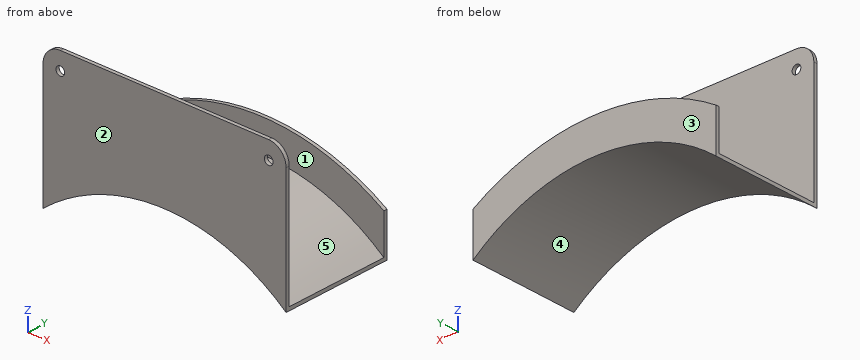
```python
from build123d import *

# Parameters (mm, degrees)
F1_DEPTH = 1.27
F3_DEPTH = 38.1
F5_DEPTH = 1.27
F6_R     = 1.5875
F7_DEPTH = 25.4


with BuildPart() as f1:
    # F0 (on Front) → F1 (new body)
    with BuildSketch(Plane.XZ):
        with BuildLine():
            Line((-44.45, 15.644758), (-44.45, 0))
            ThreePointArc((-44.45, 0), (0, 15.875), (44.45, 0))
            Line((44.45, 0), (44.45, 15.644758))
            ThreePointArc((44.45, 15.644758), (0, 28.575), (-44.45, 15.644758))
        make_face()
    extrude(amount=F1_DEPTH)

    # F2 (on face) → F3 (join)
    with BuildSketch(Plane.XZ.offset(1.27)):
        with BuildLine():
            ThreePointArc((-44.45, 0), (0, 15.875), (44.45, 0))
            Line((44.45, 0), (44.45, 1.27))
            ThreePointArc((44.45, 1.27), (0, 16.862218), (-44.45, 1.27))
            Line((-44.45, 1.27), (-44.45, 0))
        make_face()
    extrude(amount=F3_DEPTH)

    # F4 (on face) → F5 (join)
    with BuildSketch(Plane.XZ.offset(39.37)):
        with BuildLine():
            Line((-44.45, 44.45), (-44.45, 0))
            ThreePointArc((-44.45, 0), (0, 15.875), (44.45, 0))
            Line((44.45, 0), (44.45, 44.45))
            ThreePointArc((44.45, 44.45), (42.590128, 48.940128), (38.1, 50.8))
            Line((38.1, 50.8), (-38.1, 50.8))
            ThreePointArc((-38.1, 50.8), (-42.590128, 48.940128), (-44.45, 44.45))
        make_face()
    extrude(amount=F5_DEPTH)

    # F6 (on face) → F7 (cut)
    with BuildSketch(Plane(origin=(0, -39.37, 0), x_dir=(-1, 0, 0), z_dir=(0, 1, 0))):
        with Locations((-38.1, 44.45)):
            Circle(F6_R)
        with Locations((38.1, 44.45)):
            Circle(F6_R)
    extrude(amount=-F7_DEPTH, mode=Mode.SUBTRACT)


solid = f1.part
```
The model under review builds one solid part; all positions refer to its coordinate system, in mm. Face numbers are marked on the shaded views. A direction names the side the tool comes from. Round coordinates to 2 decimals unless told otherwise and drop trailing zeros. Write each loop counter-clockwise with the first axis right and the second up, starting at its lowest first coordinate (ties: lowest second). Pieces come first, ordered by that corner, then holes.
(1) We need section D-D on z = 18. Give the boundary of the cut face in (x, y).
(2) Machinability: for the marked faces 1 and 2, which of the approach directions +Z, -Z, +X, -X, +Y, -Y give a long, thin tool a straight path to every point of the face, cutting with its end or side? Answer none if there is none.
(3) We need section C-C on x = -30.5. Give the boundary of the cut face in (y, z).
(4) We need section A-A on z = 8. Give the boundary of the cut face in (x, y), and give its area (3 significant figures).
(5) Mouldability with a two-part tool opening along X and no side actions: class the marked faces 3, 4 and 5 as +X half, -X half, draft (parallel to the pull), parting line (faces both ways), or undercut.
(6) Wall thickness on L1, parallel to Y at x = 3.5, z = 22.5; L2, parallel to X at y = -40, z = 44; L3, parallel to Y at x = -22, z = 41: over which ranges is each line inside the solid? List them lowest first.
(7) Insertion check: pin 1 (5 mm diameter, centred on x = -38.1, z = 44.45, fed in from +Y); pin 2 (4 mm diameter, centred on x = -34.5, y = -25.5, fed in from -Z); pin 3 (5 mm diameter, centred on x = 21.5, y = -28.5, fed in from -Z). Each pin has a flat end and moves straight along its axis. Give the tip position at first contact, or say it passes through.
Findings below:
1. outline: (-44.45, -40.64) - (44.45, -40.64) - (44.45, -39.37) - (-44.45, -39.37) - close; (-40.51, -1.27) - (40.51, -1.27) - (40.51, 0) - (-40.51, 0) - close
2. face 1: +Z
2. face 2: +Z, -Z, +X, -X, -Y
3. outline: (-40.64, 8.9) - (0, 8.9) - (0, 22.76) - (-1.27, 22.76) - (-1.27, 9.99) - (-39.37, 9.99) - (-39.37, 50.8) - (-40.64, 50.8) - close
4. outline: (-44.45, -40.64) - (-32.3, -40.64) - (-32.3, 0) - (-44.45, 0) - (-44.45, -1.27) - (-34.39, -1.27) - (-34.39, -39.37) - (-44.45, -39.37) - close; (32.3, -40.64) - (44.45, -40.64) - (44.45, -39.37) - (34.39, -39.37) - (34.39, -1.27) - (44.45, -1.27) - (44.45, 0) - (32.3, 0) - close
4. area: 221 mm2
5. face 3: draft
5. face 4: undercut
5. face 5: parting line
6. L1: y = -40.64 to -39.37, -1.27 to 0
6. L2: x = -44.45 to -39.62, -36.58 to 36.58, 39.62 to 44.45
6. L3: y = -40.64 to -39.37
7. pin 1: stops at y = -39.37
7. pin 2: stops at z = 5.63
7. pin 3: stops at z = 11.64
